Solid Edge part; units mm, degrees
sketch "Sketch1" plane through (0, 0, 0) normal (1, 0, 0) x (0, 1, 0)
  line L0 (0, 0) -> (10, 0)
  line L1 (10, 0) -> (10, -9.7)
  line L2 (10, -9.7) -> (8.65, -9.7)
  line L3 (8.65, -9.7) -> (8.65, -146.3)
  line L4 (8.65, -146.3) -> (10, -146.3)
  line L5 (10, -146.3) -> (10, -168)
  line L6 (10, -168) -> (0, -168)
  line L7 (0, -168) -> (0, 0)
revolve "RevolvedProtrusion1" add sketch "Sketch1" angle 360 about axis through (0, 0, -168) along (0, 0, 1)
sketch "Sketch2" plane through (0, 0, 0) normal (1, 0, 0) x (0, 1, 0)
  arc A0 (0, -168) -> (6.9282, -164) centre (0, -160) ccw
  line L0 (6.9282, -164) -> (13.8564, -152)
  line L1 (13.8564, -152) -> (17, -152)
  line L2 (17, -152) -> (17, -169)
  line L3 (17, -169) -> (0, -169)
  line L4 (0, -169) -> (0, -168)
revolve "RevolvedCutout1" cut sketch "Sketch2" angle 360 about axis through (0, 0, -169) along (0, 0, 1)
sketch "Sketch3" plane through (0, 0, 0) normal (0, -1, 0) x (1, 0, 0)
  line L0 (-20, -173) -> (-20, -150)
  line L1 (-20, -150) -> (-6.75, -150)
  arc A0 (-6.75, -150) -> (-5.95, -150.8) centre (-6.75, -150.8) cw
  line L2 (-5.95, -150.8) -> (-5.95, -171)
  line L3 (-5.95, -171) -> (5.95, -171)
  line L4 (5.95, -171) -> (5.95, -150.8)
  arc A1 (5.95, -150.8) -> (6.75, -150) centre (6.75, -150.8) cw
  line L5 (6.75, -150) -> (20, -150)
  line L6 (20, -150) -> (20, -173)
  line L7 (20, -173) -> (-20, -173)
extrude "ExtrudedCutout_1" cut sketch "Sketch3" against normal blind 10 and the other way blind 10
sketch "Sketch4" plane through (0, 0, 0) normal (0, 0, 1) x (1, 0, 0)
  line L0 (-12, -12) -> (12, -12)
  line L1 (12, -12) -> (12, 12)
  line L2 (12, 12) -> (-12, 12)
  line L3 (-12, 12) -> (-12, -12)
  line L4 (-11, -9) -> (11, -9)
  line L5 (11, -9) -> (11, 9)
  line L6 (11, 9) -> (-11, 9)
  line L7 (-11, 9) -> (-11, -9)
extrude "ExtrudedCutout_2" cut sketch "Sketch4" against normal blind 168
sketch "Sketch5" plane through (0, 0, 0) normal (0, -1, 0) x (1, 0, 0)
  line L0 (-5.95, -160) -> (-5.95, -163.5774)
  line L1 (-5.95, -163.5774) -> (-4.95, -163)
  line L2 (-4.95, -163) -> (4.95, -163)
  line L3 (4.95, -163) -> (5.95, -163.5774)
  line L4 (5.95, -163.5774) -> (5.95, -160)
  line L5 (5.95, -160) -> (-5.95, -160)
revolve "RevolvedCutout2" cut sketch "Sketch5" angle 360 about axis through (5.95, 0, -160) along (-1, 0, 0)
sketch "Sketch6" plane through (0, 0, 0) normal (1, 0, 0) x (0, 1, 0)
  line L0 (-3.1934, -150) -> (-2, -147.933)
  line L1 (-2, -147.933) -> (8.567, -147.933)
  line L2 (8.567, -147.933) -> (9, -147.5)
  line L3 (9, -147.5) -> (9, -150)
  line L4 (9, -150) -> (-3.1934, -150)
revolve "RevolvedCutout3" cut sketch "Sketch6" angle 360 about axis through (0, 9, -150) along (0, -1, 0)
sketch "Sketch7" plane through (0, 0, 0) normal (1, 0, 0) x (0, 1, 0)
  line L0 (-3.1934, -6) -> (-2, -3.933)
  line L1 (-2, -3.933) -> (8.567, -3.933)
  line L2 (8.567, -3.933) -> (9, -3.5)
  line L3 (9, -3.5) -> (9, -6)
  line L4 (9, -6) -> (-3.1934, -6)
revolve "RevolvedCutout4" cut sketch "Sketch7" angle 360 about axis through (0, 9, -6) along (0, -1, 0)
sketch "Sketch8" plane through (0, 0, 0) normal (1, 0, 0) x (0, 1, 0)
  line L0 (0, 18) -> (7, 18)
  line L1 (7, 18) -> (7, 15.5)
  line L2 (7, 15.5) -> (7.08, 15.5)
  line L3 (7.08, 15.5) -> (8, 14.58)
  line L4 (8, 14.58) -> (8, 0)
  line L5 (8, 0) -> (0, 0)
  line L6 (0, 0) -> (0, 18)
revolve "RevolvedProtrusion2" add sketch "Sketch8" angle 360 about axis through (0, 0, 0) along (0, 0, 1)
sketch "Sketch9" plane through (0, 0, 18) normal (0, 0, 1) x (1, 0, 0)
  line L0 (-10, -4.5) -> (-10, -10)
  line L1 (-10, -10) -> (10, -10)
  line L2 (10, -10) -> (10, -4.5)
  line L3 (10, -4.5) -> (3.2, -4.5)
  line L4 (3.2, -4.5) -> (3.2, -3.9067)
  arc A0 (3.2, -3.9067) -> (3.2, 3.9067) centre (0, 0) ccw
  line L5 (3.2, 3.9067) -> (3.2, 4.5)
  line L6 (3.2, 4.5) -> (10, 4.5)
  line L7 (10, 4.5) -> (10, 10)
  line L8 (10, 10) -> (-10, 10)
  line L9 (-10, 10) -> (-10, 4.5)
  line L10 (-10, 4.5) -> (-3.2, 4.5)
  line L11 (-3.2, 4.5) -> (-3.2, 3.9067)
  arc A1 (-3.2, 3.9067) -> (-3.2, -3.9067) centre (0, 0) ccw
  line L12 (-3.2, -3.9067) -> (-3.2, -4.5)
  line L13 (-3.2, -4.5) -> (-10, -4.5)
extrude "ExtrudedCutout_3" cut sketch "Sketch9" against normal blind 2.5
sketch "Sketch10" plane through (0, 0, 0) normal (1, 0, 0) x (0, 1, 0)
  line L0 (0, 18) -> (3, 18)
  line L1 (3, 18) -> (3, -24.2)
  line L2 (3, -24.2) -> (8, -24.2)
  line L3 (8, -24.2) -> (8, -129.5333)
  line L4 (8, -129.5333) -> (0, -129.5333)
  line L5 (0, -129.5333) -> (0, 18)
revolve "RevolvedCutout5" cut sketch "Sketch10" angle 360 about axis through (0, 0, -129.5333) along (0, 0, 1)
properties part number "BumbleB0480"
Can you work these out from the model? Positions are in its coordinate system, mm. A direction names the side the tool comes from. Coordinates: 2 decimals unless noted, no trailing zeros. Loops run counter-clockwise (first coordinate to the right, second up) from the corner with the lowest first, then second, coordinate; pieces in that order, holes last. Notation, with made-up numbers: (-39.75, -26) - (6.25, -26) arc R18 ccw to (6.25, 5) - close; hole circle Ø2 at (72, 15). An arc over 180 degrees is marked (long way). Answer as a JSON object with one key per item and string values. Group by question number.
Item 1: For pin 1 (1 mm diameter, centred on x = -8, y = -2.5, fed in from -Z); pin 2 (8 mm diameter, centred on x = 0, y = 0, fed in from +Z); pin 3 (1 mm diameter, centred on x = 4, z = -83, fed in from -Y); pin 4 (5 mm diameter, centred on x = 2, y = 3, fed in from +Z), each with a flat end and sliding along its axis, tell me the tip position at first contact or that it passes through.
Item 2: If we section it at C-C (z = -134.5): List the corners of the cut face in (x, y) for me.
Item 3: If we mould it in two halves opening along Y, with no side actions, what happens to faces 1 (the face through (0.07, 0.9, -162.86)), 2 (the face through (5.95, 0, -155)), 3 (the face through (0, 9, -3))? For each: released by +Y, released by -Y, zero draft, split by the parting line, or undercut.
Item 4: If we section it at A-A (y = 0): State how many separate pieces and enclosed holes the cut face has, plus the area to 3 significant figures.
Item 5: If I drill on L1, parallel to Y at x = 0.25, z = -70; L2, parallel to Z at x = -4.5, y = 0; L3, parallel to Y at x = 7, z = -73, over which ranges is the centre line in solid material (lowest first)? Write a range as from..to.
Item 6: If we section it at B-B (z = -33.5): List the corners of the cut face in (x, y) for me.
Item 7: On a 3-axis mill with a long thin cutter (end or side, diameter ignored), from which of +Z, -Z, +X, -X, +Y, -Y can I reach the whole of each face in a straight line? I mean faces 4 (the face through (0, -3, -5)), 5 (the face through (0.62, 3.36, -148.03)), 6 (the face through (-0.1, 3.4, -24.2)), 7 (the face through (-5.95, 0, -156)), 8 (the face through (8, 0, -150)). Say none if no direction works.
Returned:
{
 "1": {"pin 1": "stops at z = -150", "pin 2": "stops at z = 15.5", "pin 3": "stops at y = -7.91", "pin 4": "stops at z = 18"},
 "2": {"outline": "circle Ø17.3 at (0, 0)"},
 "3": {"face 1": "undercut", "face 2": "zero draft", "face 3": "released by +Y"},
 "4": {"separate pieces": "2", "enclosed holes": "1", "area": "1,080 mm²"},
 "5": {"L1": "y = -8.65..-8, 8..8.65", "L2": "z = -166.61..-163, -157..-129.53, -24.2..15.5", "L3": "y = -5.08..-3.87, 3.87..5.08"},
 "6": {"outline": "circle Ø17.3 at (0, 0); hole circle Ø16 at (0, 0)"},
 "7": {"face 4": "+Z", "face 5": "+Y", "face 6": "none", "face 7": "-Z, -X, +Y, -Y", "face 8": "-Z, +X, +Y, -Y"}
}
